The model under review builds one solid part; all positions refer to its coordinate system, in mm. A direction names the side the tool comes from. Give positions to 0.01 mm unless a question says otherwise; leave off trailing zeros. Order: outer loops, then holes, each group sorted by start corner. A loop starts at its lowest first (then second) coordinate and runs counter-clockwise, first axis right, second up. Notation, with made-up numbers: (5.5, -29) - (38.5, -29) arc R19 ccw to (38.5, 4) - close; hole circle Ø11 at (51.5, -4). An arc over 180 degrees is marked (long way). Use CSV: the item, a comma, the result in double quotes.
```python
from build123d import *

# Parameters (mm, degrees)
CROQUIS1_W              = 209.55
CROQUIS1_H              = 146.05
SALIENTE_EXTRUIR1_DEPTH = 3.1242
CROQUIS2_R              = 1.3335
CORTAR_EXTRUIR1_DEPTH   = 128.750584639
CROQUIS9_R              = 1.27
CORTAR_EXTRUIR6_DEPTH   = 128.750584639
CORTAR_EXTRUIR2_DEPTH   = 128.750584639
CROQUIS5_R              = 1.651
DRIVER_DEPTH            = 128.750584639
CROQUIS6_R              = 1.651
RASPI_DEPTH             = 128.750584639
CROQUIS8_R              = 1.27
CORTAR_EXTRUIR5_DEPTH   = 128.750584639
CROQUIS7_R              = 1.5875
CROQUIS7_W              = 11.1125
CROQUIS7_H              = 2.9972
CORTAR_EXTRUIR7_DEPTH   = 128.750584639
CROQUIS10_R             = 1.651
CROQUIS10_W             = 22.479
CROQUIS10_H             = 11.7856
CORTAR_EXTRUIR10_DEPTH  = 128.750584639


with BuildPart() as part:
    # Croquis1 → Saliente-Extruir1 (new body)
    with BuildSketch(Plane.XY):
        Rectangle(CROQUIS1_W, CROQUIS1_H)
    extrude(amount=SALIENTE_EXTRUIR1_DEPTH)

    # Croquis2 → Cortar-Extruir1 (cut, through all)
    with BuildSketch(Plane.XY.offset(3.1242)):
        with BuildLine():
            ThreePointArc((80.9879, 60.7314), (80.336840382, 61.877042778), (79.0194, 61.904002767))
            Line((79.0194, 61.904002767), (79.0194, 59.558797233))
            ThreePointArc((79.0194, 59.558797233), (80.336840382, 59.585757222), (80.9879, 60.7314))
        make_face()
        with BuildLine():
            Line((79.0194, 59.558797233), (79.0194, 61.904002767))
            ThreePointArc((79.0194, 61.904002767), (78.3209, 60.7314), (79.0194, 59.558797233))
        make_face()
        with Locations(Location((79.6544, -60.7314, 0), (0, 0, 180))):
            Circle(CROQUIS2_R)
    extrude(amount=-CORTAR_EXTRUIR1_DEPTH, mode=Mode.SUBTRACT)

    # Croquis9 → Cortar-Extruir6 (cut, through all)
    with BuildSketch(Plane.XY.offset(3.1242)):
        with Locations((64.9859, 37.6809)):
            Circle(CROQUIS9_R)
        with Locations((94.3229, 37.6809)):
            Circle(CROQUIS9_R)
        with Locations(Location((94.3229, -37.6809, 0), (0, 0, 180))):
            Circle(CROQUIS9_R)
        with Locations(Location((64.9859, -37.6809, 0), (0, 0, 180))):
            Circle(CROQUIS9_R)
    extrude(amount=-CORTAR_EXTRUIR6_DEPTH, mode=Mode.SUBTRACT)

    # Croquis3 → Cortar-Extruir2 (cut, through all)
    with BuildSketch(Plane.XY.offset(3.1242)):
        with BuildLine():
            ThreePointArc((19.05, 73.025), (23.540128061, 71.165128061), (25.4, 66.675))
            ThreePointArc((25.4, 66.675), (32.974773587, 49.782459091), (50.14595, 42.8625))
            Line((50.14595, 42.8625), (61.988875982, 42.8625))
            ThreePointArc((61.988875982, 42.8625), (71.32896295, 49.711127589), (74.8919, 60.7314))
            ThreePointArc((74.8919, 60.7314), (78.140718752, 65.246948176), (83.454703288, 63.601783453))
            ThreePointArc((83.454703288, 63.601783453), (99.303056378, 33.540057805), (104.775, 0))
            Line((104.775, 0), (104.775, 73.025))
            Line((104.775, 73.025), (19.05, 73.025))
        make_face()
        with BuildLine():
            Line((104.775, -73.025), (104.775, 0))
            ThreePointArc((104.775, 0), (99.303056378, -33.540057805), (83.454703288, -63.601783453))
            ThreePointArc((83.454703288, -63.601783453), (78.140718752, -65.246948176), (74.8919, -60.7314))
            ThreePointArc((74.8919, -60.7314), (71.32896295, -49.711127589), (61.988875982, -42.8625))
            Line((61.988875982, -42.8625), (50.14595, -42.8625))
            ThreePointArc((50.14595, -42.8625), (32.974773587, -49.782459091), (25.4, -66.675))
            ThreePointArc((25.4, -66.675), (23.540128061, -71.165128061), (19.05, -73.025))
            Line((19.05, -73.025), (104.775, -73.025))
        make_face()
        with BuildLine():
            ThreePointArc((-104.775, 63.5), (-101.985192091, 70.235192091), (-95.25, 73.025))
            Line((-95.25, 73.025), (-104.775, 73.025))
            Line((-104.775, 73.025), (-104.775, 63.5))
        make_face()
        with BuildLine():
            Line((-104.775, -73.025), (-95.25, -73.025))
            ThreePointArc((-95.25, -73.025), (-101.985192091, -70.235192091), (-104.775, -63.5))
            Line((-104.775, -63.5), (-104.775, -73.025))
        make_face()
    extrude(amount=-CORTAR_EXTRUIR2_DEPTH, mode=Mode.SUBTRACT)

    # Croquis5 → Driver (cut, through all)
    with BuildSketch(Plane.XY.offset(3.1242)):
        with BuildLine():
            Line((12.47775, -19.2786), (-18.82775, -19.2786))
            ThreePointArc((-18.82775, -19.2786), (-19.389016008, -19.511083992), (-19.6215, -20.07235))
            Line((-19.6215, -20.07235), (-19.6215, -25.8826))
            ThreePointArc((-19.6215, -25.8826), (-20.55143597, -28.12766403), (-22.7965, -29.0576))
            Line((-22.7965, -29.0576), (-24.7015, -29.0576))
            ThreePointArc((-24.7015, -29.0576), (-28.293602448, -30.545497552), (-29.7815, -34.1376))
            Line((-29.7815, -34.1376), (-29.7815, -54.991))
            ThreePointArc((-29.7815, -54.991), (-28.293602448, -58.583102448), (-24.7015, -60.071))
            Line((-24.7015, -60.071), (-22.7965, -60.071))
            ThreePointArc((-22.7965, -60.071), (-20.55143597, -61.00093597), (-19.6215, -63.246))
            Line((-19.6215, -63.246), (-19.6215, -69.05625))
            ThreePointArc((-19.6215, -69.05625), (-19.389016008, -69.617516008), (-18.82775, -69.85))
            Line((-18.82775, -69.85), (12.47775, -69.85))
            ThreePointArc((12.47775, -69.85), (13.039016008, -69.617516008), (13.2715, -69.05625))
            Line((13.2715, -69.05625), (13.2715, -59.563))
            ThreePointArc((13.2715, -59.563), (14.350225725, -56.958725725), (16.9545, -55.88))
            Line((16.9545, -55.88), (19.05, -55.88))
            ThreePointArc((19.05, -55.88), (20.172532015, -55.415032015), (20.6375, -54.2925))
            Line((20.6375, -54.2925), (20.6375, -34.8361))
            ThreePointArc((20.6375, -34.8361), (20.172532015, -33.713567985), (19.05, -33.2486))
            Line((19.05, -33.2486), (16.9545, -33.2486))
            ThreePointArc((16.9545, -33.2486), (14.350225725, -32.169874275), (13.2715, -29.5656))
            Line((13.2715, -29.5656), (13.2715, -20.07235))
            ThreePointArc((13.2715, -20.07235), (13.039016008, -19.511083992), (12.47775, -19.2786))
        make_face()
        with Locations((17.0815, -24.7396)):
            Circle(CROQUIS5_R)
        with Locations((-23.0505, -24.6126)):
            Circle(CROQUIS5_R)
        with Locations(Location((17.0815, -64.389, 0), (0, 0, 180))):
            Circle(CROQUIS5_R)
        with Locations(Location((-23.0505, -64.516, 0), (0, 0, 180))):
            Circle(CROQUIS5_R)
    extrude(amount=-DRIVER_DEPTH, mode=Mode.SUBTRACT)

    # Croquis6 → RasPi (cut, through all)
    with BuildSketch(Plane.XY.offset(3.1242)):
        with Locations((-29.95, 48.8814)):
            Circle(CROQUIS6_R)
        with Locations((19.05, 48.8814)):
            Circle(CROQUIS6_R)
        with Locations((19.05, -9.1186)):
            Circle(CROQUIS6_R)
        with Locations((-29.95, -9.1186)):
            Circle(CROQUIS6_R)
    extrude(amount=-RASPI_DEPTH, mode=Mode.SUBTRACT)

    # Croquis8 → Cortar-Extruir5 (cut, through all)
    with BuildSketch(Plane.XY.offset(3.1242)):
        with Locations((-95.885, 61.138037406)):
            Circle(CROQUIS8_R)
        with Locations((-68.495218831, 33.748256237)):
            Circle(CROQUIS8_R)
    extrude(amount=-CORTAR_EXTRUIR5_DEPTH, mode=Mode.SUBTRACT)

    # Croquis7 → Cortar-Extruir7 (cut, through all)
    with BuildSketch(Plane.XY.offset(3.1242)):
        with Locations((-92.508859415, -66.7639)):
            Circle(CROQUIS7_R)
        with Locations((-71.871359415, -66.7639)):
            Circle(CROQUIS7_R)
        with Locations((-82.190109415, -66.7639)):
            Rectangle(CROQUIS7_W, CROQUIS7_H)
    extrude(amount=-CORTAR_EXTRUIR7_DEPTH, mode=Mode.SUBTRACT)

    # Croquis10 → Cortar-Extruir10 (cut, through all)
    with BuildSketch(Plane.XY.offset(3.1242)):
        with Locations((82.0039, 9.652)):
            Circle(CROQUIS10_R)
        with Locations((82.0039, 0)):
            Rectangle(CROQUIS10_W, CROQUIS10_H)
        with Locations((82.0039, -9.652)):
            Circle(CROQUIS10_R)
    extrude(amount=-CORTAR_EXTRUIR10_DEPTH, mode=Mode.SUBTRACT)


solid = part.part
```
Item 1: Mouldability with a two-part tool opening along Y and no side actions: class faces 1 (the face through (-102.06, 70.16, 1.58)), 2 (the face through (-28.333, -58.543, 1.584)), 3 (the face through (-1, 1, 3.124)) as pulls with the +Y half, pulls with the -Y half, needs draft (parallel to the pull), parting line crosses it, or undercut.
Results list:
face 1,"pulls with the +Y half"
face 2,"undercut"
face 3,"needs draft"
Item 2: Take a section at B-B, the plane y = 29.5. Give the boundary of the cut face in (x, z) (3 decimals).
Results list:
outline,"(-104.775, 0) - (100.568, 0) - (100.568, 3.124) - (-104.775, 3.124) - close"
Item 3: Tool access review of faces 4 (the face through (23.49, 71.214, 1.584)), 5 (the face through (32.78, 49.97, 1.58)), 6 (the face through (-28.254, -30.506, 1.584)), 7 (the face through (71.425, -49.845, 1.584)), 8 (the face through (23.589, -71.115, 1.584)): name each direction out of +Z, -Z, +X, -X, +Y, -Y from which nothing blocks a thin tool from reaching the whole face with its end or side.
Results list:
face 4,"+Z, -Z, +X, +Y"
face 5,"+Z, -Z, +Y"
face 6,"+Z, -Z"
face 7,"+Z, -Z, -Y"
face 8,"+Z, -Z, +X, -Y"
Item 4: Take a section at C-C, the plane z = 0.7. State how many separate pieces and enclosed holes the cut face has, and give its area (3 significant figures).
Results list:
separate pieces,"1"
enclosed holes,"23"
area,"24,000 mm2"
Item 5: Take a section at A-A, the plane x = -14.5. Give the boundary of the cut face in (y, z) (3 decimals), and give its area (3 significant figures).
Results list:
outline,"(-73.025, 0) - (-69.85, 0) - (-69.85, 3.124) - (-73.025, 3.124) - close; (-19.279, 0) - (73.025, 0) - (73.025, 3.124) - (-19.279, 3.124) - close"
area,"298 mm2"
Item 6: Clearance check with flat-ended pins moving along their axes: pin 1 (1.6 mm diameter, centred on y = -46, z = 1.5, fed in from +X); pin 2 (0.9 mm diameter, centred on y = -66.5, z = 2, fed in from -X). State where each tip first meets the part, or that it passes through.
Results list:
pin 1,"stops at x = 94.6"
pin 2,"stops at x = -104.43"
Item 7: Wall thickness on L1, parallel to Y at x = 19.05, z = 1.8 (3 decimals); L2, parallel to Y at x = -29.95, z = 2.4 (3 decimals); L3, parallel to Y at x = -86, z = 1.6 (1 decimal): over which ranges is each line inside the solid? List them lowest first.
Results list:
L1,"y = -73.025 to -55.88, -33.249 to -10.77, -7.468 to 47.23, 50.532 to 73.025"
L2,"y = -73.025 to -10.77, -7.468 to 47.23, 50.532 to 73.025"
L3,"y = -73 to -68.3, -65.3 to 73"
